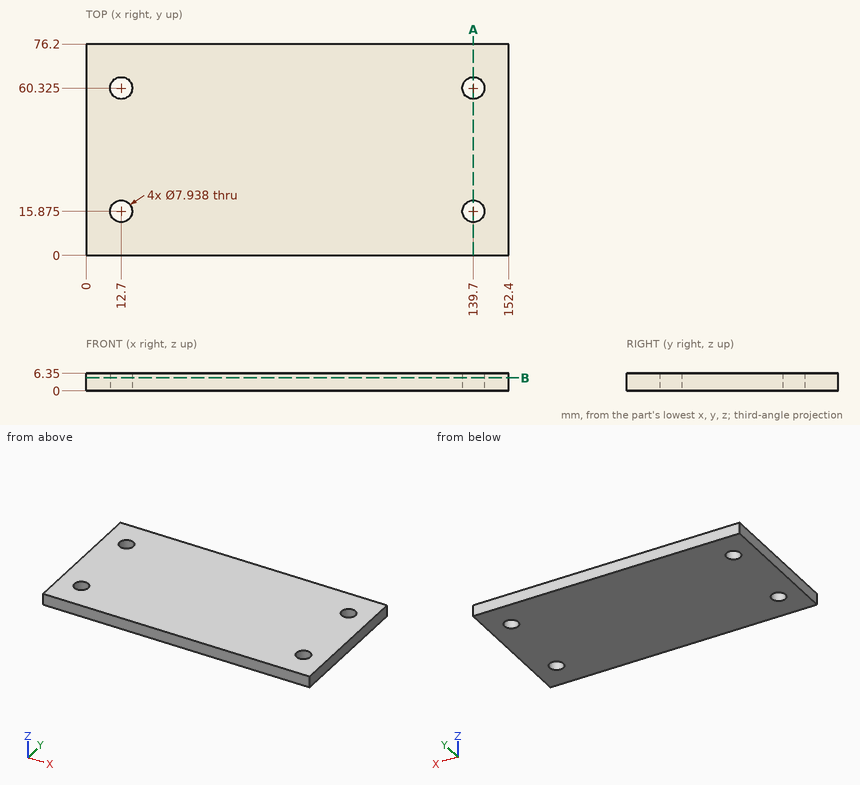
The figure shows three views and two pictorial views of one solid part (mm, origin at its lowest corner). Answer the questions. Give positions to 0.01 mm unless a question says otherwise; leave off trailing zeros. Write each loop counter-clockwise with the first axis right and the second up, starting at its lowest first coordinate (ties: lowest second). Pieces come first, ordered by that corner, then holes. Notation, with made-up numbers: (64, 31) -> (91, 31) arc R7 ccw to (91, 40) -> close; hole circle Ø2 at (61, 65.5). An arc over 180 degrees is marked (long way). Write each question's results on one line, items separated by ' | '.
1. This flat-tipped pin is pushed along its axis until it touches: pin 1 Ø7 at (x, y) = (139.7, 15.875) entering from -Z. Where does it stop, or does it pass through?
Data:
pin 1: through
2. Find section A-A on x = 139.7. Determine the outline of the cut face in (y, z).
Data:
outline: (0, 0) -> (11.91, 0) -> (11.91, 6.35) -> (0, 6.35) -> close; (19.84, 0) -> (56.36, 0) -> (56.36, 6.35) -> (19.84, 6.35) -> close; (64.29, 0) -> (76.2, 0) -> (76.2, 6.35) -> (64.29, 6.35) -> close
3. Find section B-B on z = 4.75. Determine the outline of the cut face in (x, y) (1 decimal), and give its area (3 significant figures).
Data:
outline: (0, 0) -> (152.4, 0) -> (152.4, 76.2) -> (0, 76.2) -> close; hole circle Ø7.9 at (12.7, 15.9); hole circle Ø7.9 at (12.7, 60.3); hole circle Ø7.9 at (139.7, 15.9); hole circle Ø7.9 at (139.7, 60.3) | area: 11,400 mm^2
4. Straight lines are drawn through the part: L1, parallel to Y at x = 139.7, z = 2.5; L2, parallel to X at y = 13.5, z = 3.5; L3, parallel to X at y = 59.5, z = 0.75. For each, find the intervals that lie inside material, in ascending order.
Data:
L1: 0 to 11.91, 19.84 to 56.36, 64.29 to 76.2 | L2: 0 to 9.52, 15.88 to 136.52, 142.88 to 152.4 | L3: 0 to 8.82, 16.58 to 135.82, 143.58 to 152.4
